Build history of the part. All positions in model axes, mm. Face numbers are marked on the shaded views. A direction names the side the tool comes from. Round coordinates to 2 decimals unless told otherwise and drop trailing zeros. Loops run counter-clockwise (first coordinate to the right, second up) from the corner with the lowest first, then second, coordinate; pieces in that order, holes last. Notation, with made-up numbers: (73.5, 72) - (89.5, 72) arc R14 ccw to (89.5, 84) - close; hole circle Ø2 at (-16, -6.75). An arc over 180 degrees is marked (long way). Put each result on its own line as item: value. Start each with the question number.
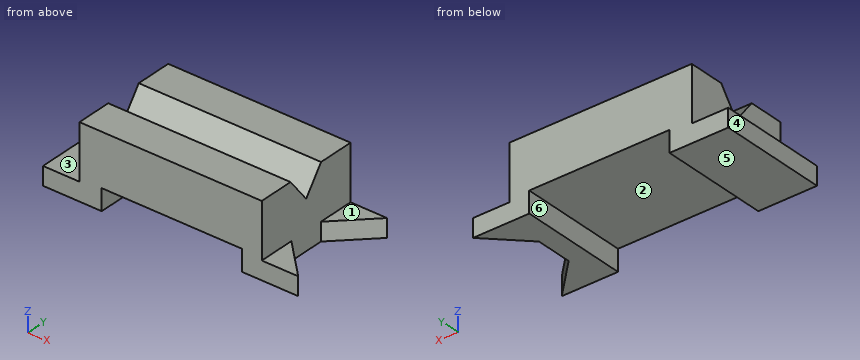
from build123d import *

# Parameters (mm, degrees)
F0_W      = 152.4
F0_H      = 76.2
F1_DEPTH  = 50.8
F3_DEPTH  = 50.801
F4_DEPTH  = 38.1
F5_DEPTH  = 38.1
F7_DEPTH  = 127.001
F8_W      = 97.740334
F8_H      = 14.750447
F9_DEPTH  = 76.201
F10_W     = 76.2
F10_H     = 12.7
F11_DEPTH = 25.4


with BuildPart() as f1:
    # F0 (on Top) → F1 (new body)
    with BuildSketch(Plane.XY):
        with Locations((2.035878, 0)):
            Rectangle(F0_W, F0_H)
    extrude(amount=F1_DEPTH)

    # F2 (on face) → F3 (cut, through all)
    with BuildSketch(Plane.XY.offset(50.8)):
        Polygon((78.235878, -38.1), (78.235878, 38.1), (52.835878, 12.7), (52.835878, -12.7), align=None)
    extrude(amount=-F3_DEPTH, mode=Mode.SUBTRACT)

    # F2 (on face) → F4 (cut)
    with BuildSketch(Plane.XY.offset(50.8)):
        Polygon((52.835878, 12.7), (78.235878, 38.1), (52.835878, 38.1), align=None)
    extrude(amount=-F4_DEPTH, mode=Mode.SUBTRACT)

    # F2 (on face) → F5 (cut)
    with BuildSketch(Plane.XY.offset(50.8)):
        Polygon((52.835878, -38.1), (78.235878, -38.1), (52.835878, -12.7), align=None)
    extrude(amount=-F5_DEPTH, mode=Mode.SUBTRACT)

    # F6 (on face) → F7 (cut, through all)
    with BuildSketch(Plane.YZ.offset(52.835878)):
        Polygon((12.813521, 50.8), (-13.409496, 50.8), (0, 33.523746), align=None)
    extrude(amount=-F7_DEPTH, mode=Mode.SUBTRACT)

    # F8 (on face) → F9 (cut, through all)
    with BuildSketch(Plane.XZ.offset(38.1)):
        with Locations((-9.811988, 7.375223)):
            Rectangle(F8_W, F8_H)
    extrude(amount=-F9_DEPTH, mode=Mode.SUBTRACT)

    # F10 (on face) → F11 (join)
    with BuildSketch(Plane(origin=(-74.164122, 0, 0), x_dir=(0, -1, 0), z_dir=(-1, 0, 0))):
        with Locations((0, 6.35)):
            Rectangle(F10_W, F10_H)
    extrude(amount=F11_DEPTH)


solid = f1.part
1) Slice it at B-B, the plane x = -6. Write the cut outline in (y, z), and give its area (3 significant figures).
2) Drop flat-ended pins along their axis: pin 1 Ø16 at (y, z) = (13.5, 6) entering from +X; pin 2 Ø1.5 at (y, z) = (-6, 23) entering from +X; pin 3 Ø12 at (y, z) = (28.5, 40.5) entering from -X. Give the stop position or say it passes through.
3) Slice it at D-D, the plane z = 8. Write the cut outline in (x, y), and give its area (3 significant figures).
4) Which spindle directions (+Z, -Z, +X, -X, +Y, -Y) get a long thin tool onto all of the face, cutting with end or side? Do the marked faces 1, 2 and 3. Say none if no direction does.
5) Drill centre lines: line 1 (X direction, y = 10, z = 2.5); line 2 (Z direction, x = -34, y = 14); line 3 (X direction, y = -9, z = 25.5). Where is each one in solid material? Low to high. Write a range as [from, to].
6) Slice it at A-A, the plane z = 47.5. Write the cut outline in (x, y), and give its area (3 significant figures).
7) Slice it at C-C, the plane y = 10. Write the cut outline in (x, z), and give its area (3 significant figures).
8) Pull direction X, two halves, no side cores. Call the marked faces 4, 5 and 6: pulls with the +X half, pulls with the -X half, needs draft (parallel to the pull), parting line crosses it, or undercut.
Taken from the geometry:
1. outline: (-38.1, 14.75) - (38.1, 14.75) - (38.1, 50.8) - (12.81, 50.8) - (0, 33.52) - (-13.41, 50.8) - (-38.1, 50.8) - close
1. area: 2,520 mm2
2. pin 1: stops at x = 61.64
2. pin 2: stops at x = 52.84
2. pin 3: stops at x = -74.16
3. outline: (-99.56, -38.1) - (-58.68, -38.1) - (-58.68, 38.1) - (-99.56, 38.1) - close; (39.06, -38.1) - (78.24, -38.1) - (52.84, -12.7) - (52.84, 12.7) - (78.24, 38.1) - (39.06, 38.1) - close
3. area: 4,810 mm2
4. face 1: +Z, +X, +Y, -Y
4. face 2: -Z, +Y, -Y
4. face 3: +Z, -X, +Y, -Y
5. line 1: x = [-99.56, -58.68], [39.06, 52.84]
5. line 2: z = [14.75, 50.8]
5. line 3: x = [-74.16, 52.84]
6. outline: (-74.16, -38.1) - (52.84, -38.1) - (52.84, -10.85) - (-74.16, -10.85) - close; (-74.16, 10.37) - (52.84, 10.37) - (52.84, 38.1) - (-74.16, 38.1) - close
6. area: 6,980 mm2
7. outline: (-99.56, 0) - (-58.68, 0) - (-58.68, 14.75) - (39.06, 14.75) - (39.06, 0) - (52.84, 0) - (52.84, 47.01) - (-74.16, 47.01) - (-74.16, 12.7) - (-99.56, 12.7) - close
7. area: 4,850 mm2
8. face 4: pulls with the -X half
8. face 5: needs draft
8. face 6: undercut
